The model under review builds one solid part; all positions refer to its coordinate system, in mm. A direction names the side the tool comes from. Coordinates: 2 decimals unless noted, no trailing zeros. Order: outer loops, then holes, each group sorted by start corner. A loop starts at its lowest first (then second) coordinate and runs counter-clockwise, first axis right, second up. Notation, with made-up numbers: (9.5, -13.5) -> (63.5, -13.5) arc R18 cw to (63.5, 10.5) -> close; hole circle Ø1 at (2, -17.5). An arc over 180 degrees is marked (long way). Put each result on its own line as item: value.
from build123d import *

# Parameters (mm, degrees)
F0_R     = 33.5
F1_DEPTH = 7
F3_DEPTH = 7
F4_W     = 10
F4_H     = 85.8
F5_DEPTH = 13


with BuildPart() as f1:
    # F0 (on Top) → F1 (new body)
    with BuildSketch(Plane.XY):
        with BuildLine():
            ThreePointArc((0, -42.9), (-42.9, 0), (0, 42.9))
            Line((0, 42.9), (-55.5, 42.9))
            Line((-55.5, 42.9), (-55.5, -42.9))
            Line((-55.5, -42.9), (0, -42.9))
        make_face()
        with BuildLine():
            ThreePointArc((0, -42.9), (30.334881, -30.334881), (42.9, 0))
            ThreePointArc((42.9, 0), (30.334881, 30.334881), (0, 42.9))
            ThreePointArc((0, 42.9), (-42.9, 0), (0, -42.9))
        make_face()
        Circle(F0_R, mode=Mode.SUBTRACT)
    extrude(amount=F1_DEPTH)

    # F2 (on face) → F3 (join)
    with BuildSketch(Plane(origin=(0, 0, 0), x_dir=(1, 0, 0), z_dir=(0, 0, -1))):
        with BuildLine():
            Line((-55.5, -42.9), (0, -42.9))
            ThreePointArc((0, -42.9), (42.9, 0), (0, 42.9))
            Line((0, 42.9), (-55.5, 42.9))
            Line((-55.5, 42.9), (-55.5, -42.9))
        make_face()
    extrude(amount=F3_DEPTH)

    # F4 (on face) → F5 (join)
    with BuildSketch(Plane(origin=(0, 0, -7), x_dir=(1, 0, 0), z_dir=(0, 0, -1))):
        with Locations((-50.5, 0)):
            Rectangle(F4_W, F4_H)
    extrude(amount=F5_DEPTH)


solid = f1.part
Item 1: Consider section B-B on x = 14. Write out the cut boundary in (y, z), and give its area (3 significant figures).
Answers below:
outline: (-40.55, -7) -> (40.55, -7) -> (40.55, 7) -> (30.43, 7) -> (30.43, 0) -> (-30.43, 0) -> (-30.43, 7) -> (-40.55, 7) -> close
area: 709 mm^2
Item 2: Consider section D-D on z = -10. Write out the cut boundary in (x, y).
Answers below:
outline: (-55.5, -42.9) -> (-45.5, -42.9) -> (-45.5, 42.9) -> (-55.5, 42.9) -> close
Item 3: For pin 1 Ø2 at (y, z) = (-14.5, -10.5) entering from +X; pin 2 Ø5 at (y, z) = (-14.5, -8.5) entering from +X; pin 3 Ø5 at (y, z) = (-0.5, -8.5) entering from +X, all flat-tipped, find the tip position at first contact; note any pin that passes through.
Answers below:
pin 1: x = -45.5
pin 2: x = 41.04
pin 3: x = 42.9
Item 4: Consider section A-A on z = 3.25. Write out the cut boundary in (x, y).
Answers below:
outline: (-55.5, -42.9) -> (0, -42.9) arc R42.9 ccw to (0, 42.9) -> (-55.5, 42.9) -> close; hole circle Ø67 at (0, 0)
Item 5: Consider section C-C on y = -7.5. Write out the cut boundary in (x, z), and give its area (3 significant figures).
Answers below:
outline: (-55.5, -20) -> (-45.5, -20) -> (-45.5, -7) -> (42.24, -7) -> (42.24, 7) -> (32.65, 7) -> (32.65, 0) -> (-32.65, 0) -> (-32.65, 7) -> (-55.5, 7) -> close
area: 1,040 mm^2
Item 6: Mouldability with a two-part tool opening along X and no side actions: class faces 1 (the flat face through (0, 0, 0)), 2 (the flat face through (-55.5, 1, -6)), 3 (the flat face through (-45.5, 1, -13)) as +X half, -X half, draft (parallel to the pull), parting line (faces both ways), or undercut.
Answers below:
face 1: undercut
face 2: -X half
face 3: +X half
Item 7: For faces 4 (the cylindrical face through (-7.262, -32.703, 3.451)), 5 (the flat face through (-2, -1, -7)), 6 (the flat face through (-40, 1, 7)), list the 3-axis set-ups (+Z, -Z, +X, -X, +Y, -Y) from which the entire face can be reached by the end or side of a thin tool; tool diameter is ignored.
Answers below:
face 4: +Z
face 5: -Z, +X, +Y, -Y
face 6: +Z, +X, -X, +Y, -Y
Item 8: For line 1 (Y direction, x = 0, z = 5); line 2 (Z direction, x = -15, y = -36.5); line 3 (Z direction, x = -19, y = -2.5), list the stretches that pass through material, from the lowest coordinate up. Write a range as from..to.
Answers below:
line 1: -42.9..-33.5, 33.5..42.9
line 2: -7..7
line 3: -7..0
